The listing builds one solid part. Answer for the finished solid, in the listing's coordinates (mm). A direction names the side the tool comes from. Coordinates: 2 decimals unless noted, no trailing zeros. Order: outer loops, then holes, each group sorted by start corner. A loop starts at its lowest first (then second) coordinate and runs counter-clockwise, first axis right, second up. Notation, with made-up numbers: (82.5, -8.75) - (104.5, -8.75) arc R19 ccw to (104.5, 22.25) - close; hole circle Ø4 at (59.5, 20). An arc over 180 degrees is marked (long way). Use one line per item in the form item = value. Start each with the question number.
Item 1: Section A-A, the plane z = -3 is taken. Write down the section's boundary in (x, y), and give its area (3 significant figures).
Item 2: Section D-D, the plane z = 16 is taken. Write down the section's boundary in (x, y), and give its area (3 significant figures).
Item 3: Section C-C, the plane y = 3.9 is taken. Count the separate pieces of the cut face and the enclosed holes in it, and give its area (3 significant figures).
Item 4: Section B-B, the plane x = -10.5 is taken. Write down the section's boundary in (y, z), and give its area (3 significant figures).
Item 5: Each of these flat-tipped pins is pushed along its axis until it touches: pin 1 Ø2.5 at (y, z) = (1.5, -7) entering from -X; pin 2 Ø2.5 at (x, y) = (-22, 1.5) entering from +Z; pin 3 Ø1.5 at (x, y) = (-23.5, 2.5) entering from -Z; pin 4 Ø5 at (x, z) = (21.5, 1) entering from -Y. Where does it stop, or does it pass through?
Item 6: A tool of negligible diameter and unlimited length cuts with its end or side. For faces 4 (the flat face through (-23, 3, 12.764)), 5 (the flat face through (48, 3, 12.764)), 6 (the flat face through (3.048, 3, -1)), 7 (the flat face through (50.673, 3, -1)), from which of +Z, -Z, +X, -X, +Y, -Y can it reach the whole face along a straight path? Write none if from no direction.
Item 7: The mould has two halves that part along Z. Classify faces 1 (the flat face through (48, 3, -5.016)), 2 (the flat face through (-23, 3, -15.176)), 3 (the flat face through (12, 5.08, -6)): released by +Z, released by -Z, zero draft, split by the parting line, or undercut.
Item 8: Consider line 1 along X through (y, z) = (3.05, -1.5); line 2 along Z through (x, y) = (46.5, 3.1); line 3 along Z through (x, y) = (40, 1.7). Determine where each line is inside the solid, lowest interval first. Write a range as [from, to].
from build123d import *

# Parameters (mm, degrees)
SKETCH1_W           = 76.2
SKETCH1_H           = 38.1
BOSS_EXTRUDE1_DEPTH = 5.08
SKETCH2_W           = 5.08
SKETCH2_H           = 5.08
CUT_EXTRUDE1_DEPTH  = 5.08
SKETCH3_W           = 6.35
SKETCH3_H           = 5.08
CUT_EXTRUDE2_DEPTH  = 5.08


with BuildPart() as part:
    # Sketch1 → Boss-Extrude1 (new body)
    with BuildSketch(Plane(origin=(0, 0, 0), x_dir=(1, 0, 0), z_dir=(0, 1, 0))):
        with Locations((12.573, 1.2065)):
            Rectangle(SKETCH1_W, SKETCH1_H)
    extrude(amount=BOSS_EXTRUDE1_DEPTH)

    # Sketch2 → Cut-Extrude1 (cut)
    with BuildSketch(Plane(origin=(0, 5.08, 0), x_dir=(1, 0, 0), z_dir=(0, 1, 0))):
        with Locations((-22.987, -5.1435)):
            Rectangle(SKETCH2_W, SKETCH2_H)
        with Locations((48.133, 17.7165)):
            Rectangle(SKETCH2_W, SKETCH2_H)
        with Locations((48.133, 7.5565)):
            Rectangle(SKETCH2_W, SKETCH2_H)
        with Locations((48.133, -15.3035)):
            Rectangle(SKETCH2_W, SKETCH2_H)
        with Locations((48.133, -5.1435)):
            Rectangle(SKETCH2_W, SKETCH2_H)
        with Locations((-22.987, -15.3035)):
            Rectangle(SKETCH2_W, SKETCH2_H)
        with Locations((-22.987, 7.5565)):
            Rectangle(SKETCH2_W, SKETCH2_H)
        with Locations((-22.987, 17.7165)):
            Rectangle(SKETCH2_W, SKETCH2_H)
    extrude(amount=-CUT_EXTRUDE1_DEPTH, mode=Mode.SUBTRACT)

    # Sketch3 → Cut-Extrude2 (cut)
    with BuildSketch(Plane(origin=(0, 5.08, 0), x_dir=(1, 0, 0), z_dir=(0, 1, 0))):
        with Locations((-12.827, 1.2065)):
            Rectangle(SKETCH3_W, SKETCH3_H)
        with Locations((12.573, 1.2065)):
            Rectangle(SKETCH3_W, SKETCH3_H)
        with Locations((25.273, 1.2065)):
            Rectangle(SKETCH3_W, SKETCH3_H)
        with Locations((37.973, 1.2065)):
            Rectangle(SKETCH3_W, SKETCH3_H)
        with Locations((-0.127, 1.2065)):
            Rectangle(SKETCH3_W, SKETCH3_H)
    extrude(amount=-CUT_EXTRUDE2_DEPTH, mode=Mode.SUBTRACT)


solid = part.part
Response:
q1.outline = (-25.53, 0) - (-16, 0) - (-16, 5.08) - (-25.53, 5.08) - close; (-9.65, 0) - (-3.3, 0) - (-3.3, 5.08) - (-9.65, 5.08) - close; (3.05, 0) - (9.4, 0) - (9.4, 5.08) - (3.05, 5.08) - close; (15.75, 0) - (22.1, 0) - (22.1, 5.08) - (15.75, 5.08) - close; (28.45, 0) - (34.8, 0) - (34.8, 5.08) - (28.45, 5.08) - close; (41.15, 0) - (50.67, 0) - (50.67, 5.08) - (41.15, 5.08) - close
q1.area = 226 mm2
q2.outline = (-20.45, 0) - (45.59, 0) - (45.59, 5.08) - (-20.45, 5.08) - close
q2.area = 335 mm2
q3.separate_pieces = 1
q3.enclosed_holes = 5
q3.area = 2,540 mm2
q4.outline = (0, -20.26) - (5.08, -20.26) - (5.08, -3.75) - (0, -3.75) - close; (0, 1.33) - (5.08, 1.33) - (5.08, 17.84) - (0, 17.84) - close
q4.area = 168 mm2
q5.pin_1 = -20.45
q5.pin_2 = 12.76
q5.pin_3 = -15.18
q5.pin_4 = 0
q6.face_4 = +Z, -X, +Y, -Y
q6.face_5 = +Z, +X, +Y, -Y
q6.face_6 = +Y, -Y
q6.face_7 = +Z, -Z, +X, +Y, -Y
q7.face_1 = undercut
q7.face_2 = released by -Z
q7.face_3 = zero draft
q8.line_1 = [-25.53, -16], [-9.65, -3.3], [3.05, 9.4], [15.75, 22.1], [28.45, 34.8], [41.15, 50.67]
q8.line_2 = [-15.18, -10.1], [-5.02, 2.6], [7.68, 12.76]
q8.line_3 = [-20.26, -3.75], [1.33, 17.84]
